from build123d import *

# Parameters (mm, degrees)
SKETCH_1_R          = 4
EXTRUDE_1_DEPTH     = 1.2
CHAMFER_1_SIZE      = 0.5
SKETCH_3_R          = 2
EXTRUDE_2_DEPTH     = 8
CUT_EXTRUDE_1_DEPTH = 2.2


with BuildPart() as part:
    # 草图1 → 凸台-拉伸1 (new body)
    with BuildSketch(Plane.XY):
        Circle(SKETCH_1_R)
    extrude(amount=EXTRUDE_1_DEPTH)

    # 倒角1
    chamfer_1_edges = [part.edges().sort_by_distance(p)[0] for p in [
        (-4, 0, 0),
    ]]
    chamfer(chamfer_1_edges, length=CHAMFER_1_SIZE)

    # 草图3 → 凸台-拉伸2 (add)
    with BuildSketch(Plane.XY.offset(1.2)):
        Circle(SKETCH_3_R)
    extrude(amount=EXTRUDE_2_DEPTH)

    # 草图4 → 切除-拉伸1 (cut)
    with BuildSketch(Plane(origin=(0, 0, 0), x_dir=(-1, 0, 0), z_dir=(0, 0, -1))):
        Polygon((0, 1.443375673), (-1.25, 0.721687836), (-1.25, -0.721687836), (0, -1.443375673), (1.25, -0.721687836), (1.25, 0.721687836), align=None)
    extrude(amount=-CUT_EXTRUDE_1_DEPTH, mode=Mode.SUBTRACT)


solid = part.part
Geometry: final body of the model. Coordinates: model frame, mm. A direction names the side the tool comes from. Give positions to 0.01 mm unless a question says otherwise; leave off trailing zeros. Write each loop counter-clockwise with the first axis right and the second up, starting at its lowest first coordinate (ties: lowest second). Pieces come first, ordered by that corner, then holes. Notation, with made-up numbers: (41, 58.25) - (78, 58.25) arc R9 ccw to (78, 64.25) - close; hole circle Ø3 at (-11.75, 45). An arc over 180 degrees is marked (long way). Return JSON: item names as keys, results as strings. Group by question number.
1) First-contact query: P1, Ø0.8, axis at x = 0, y = 0, coming from the -Z side; P2, Ø1, axis at y = 2, z = 8, coming from the +X side. Flat tips, straight axial feed; report the tip coordinate or a pass-through.
2) Mould query, pull axis X, two halves, no side actions, for faces 1 (the flat face through (0, 0, 2.2)), 2 (the flat face through (-2, -1, 1.2)), 3 (the cylindrical face through (0, -2, 5)). Classes: released by +X, released by -X, zero draft, split by the parting line, or undercut.
3) Section A-A on z = 1.5. Return the cut outline in (x, y).
4) Set-up query: faces 4 (the flat face through (0, -2, 0)), 5 (the flat face through (-0.616, -1.088, 1.085)). Return all of +Z, -Z, +X, -X, +Y, -Y with unobstructed straight access to the full face (end or side cutting, diameter ignored); none if empty.
5) Section B-B on y = 0. Return the cut outline in (x, z), plus the area to 4 significant figures.
6) Line query: line 1 (Z direction, x = 0.25, y = 2.5); line 2 (Y direction, x = -0.25, z = 3.5); line 3 (Y direction, x = -0.5, z = 3.75). Output: solid intervals per line, ascending.
7) Section C-C on z = 7.25. Return the cut outline in (x, y).
Filled in:
{
 "1": {"P1": "stops at z = 2.2", "P2": "stops at x = 1.32"},
 "2": {"face 1": "undercut", "face 2": "zero draft", "face 3": "split by the parting line"},
 "3": {"outline": "circle Ø4 at (0, 0); hole (-1.25, -0.72) - (0, -1.44) - (1.25, -0.72) - (1.25, 0.72) - (0, 1.44) - (-1.25, 0.72) - close"},
 "4": {"face 4": "-Z, +X, -X, +Y, -Y", "face 5": "-Z"},
 "5": {"outline": "(-4, 0.5) - (-3.5, 0) - (-1.25, 0) - (-1.25, 2.2) - (1.25, 2.2) - (1.25, 0) - (3.5, 0) - (4, 0.5) - (4, 1.2) - (2, 1.2) - (2, 9.2) - (-2, 9.2) - (-2, 1.2) - (-4, 1.2) - close", "area": "35.85 mm^2"},
 "6": {"line 1": "z = 0 to 1.2", "line 2": "y = -1.98 to 1.98", "line 3": "y = -1.94 to 1.94"},
 "7": {"outline": "circle Ø4 at (0, 0)"}
}
